Can you work these out from the model? Positions are in its coordinate system, mm. Face numbers are marked on the shaded views. Give positions to 0.01 mm unless a question says otherwise; leave off trailing zeros. Loops run counter-clockwise (first coordinate to the right, second up) from the corner with the lowest first, then second, coordinate; pieces in that order, holes last. Notation, with made-up numbers: M 43.25,1.5 L 91.25,1.5 A31 ccw 91.25,28.5 Z; hole C -39.75,22.25 d6. An arc over 180 degrees is marked long. Answer as a JSON object with one key per item and string values.
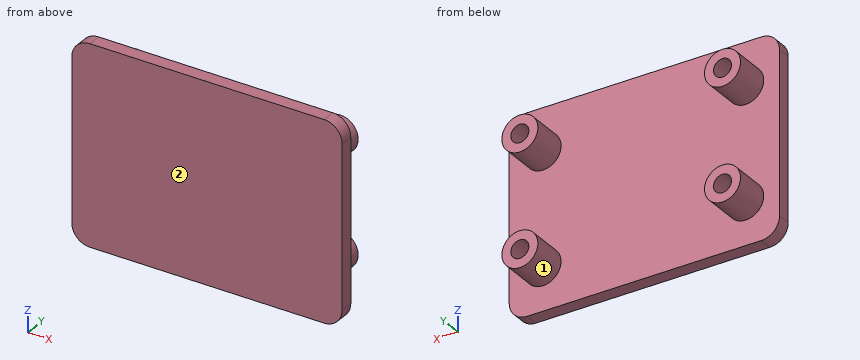
```python
from build123d import *

# Parameters (mm, degrees)
BOSS_EXTRUDE1_DEPTH = 3
SKETCH2_R           = 4
BOSS_EXTRUDE2_DEPTH = 8
SKETCH3_R           = 2
CUT_EXTRUDE1_DEPTH  = 7


with BuildPart() as part:
    # Sketch1 → Boss-Extrude1 (new body)
    with BuildSketch(Plane(origin=(0, 0, 0), x_dir=(1, 0, 0), z_dir=(0, 1, 0))):
        with BuildLine():
            Line((-26, -22), (26, -22))
            ThreePointArc((26, -22), (28.828427125, -20.828427125), (30, -18))
            Line((30, -18), (30, 18))
            ThreePointArc((30, 18), (28.828427125, 20.828427125), (26, 22))
            Line((26, 22), (-26, 22))
            ThreePointArc((-26, 22), (-28.828427125, 20.828427125), (-30, 18))
            Line((-30, 18), (-30, -18))
            ThreePointArc((-30, -18), (-28.828427125, -20.828427125), (-26, -22))
        make_face()
    extrude(amount=BOSS_EXTRUDE1_DEPTH)

    # Sketch2 → Boss-Extrude2 (add)
    with BuildSketch(Plane(origin=(0, 3, 0), x_dir=(1, 0, 0), z_dir=(0, 1, 0))):
        with Locations(Location((22.5, -12.5, 0), (0, 0, 270))):
            Circle(SKETCH2_R)
        with Locations(Location((22.5, 12.5, 0), (0, 0, 270))):
            Circle(SKETCH2_R)
        with Locations(Location((-22.5, -12.5, 0), (0, 0, 270))):
            Circle(SKETCH2_R)
        with Locations(Location((-22.5, 12.5, 0), (0, 0, 270))):
            Circle(SKETCH2_R)
    extrude(amount=BOSS_EXTRUDE2_DEPTH)

    # Sketch3 → Cut-Extrude1 (cut)
    with BuildSketch(Plane(origin=(0, 11, 0), x_dir=(1, 0, 0), z_dir=(0, 1, 0))):
        with Locations(Location((22.5, -12.5, 0), (0, 0, 270))):
            Circle(SKETCH3_R)
        with Locations(Location((22.5, 12.5, 0), (0, 0, 270))):
            Circle(SKETCH3_R)
        with Locations(Location((-22.5, -12.5, 0), (0, 0, 270))):
            Circle(SKETCH3_R)
        with Locations(Location((-22.5, 12.5, 0), (0, 0, 270))):
            Circle(SKETCH3_R)
    extrude(amount=-CUT_EXTRUDE1_DEPTH, mode=Mode.SUBTRACT)


solid = part.part
```
1) Suppose I cut it at D-D, the plane x = -6.5. Write out the boundary of the cut face in (y, z), and give its area (3 significant figures).
Answer list:
{"outline": "M 0,-22 L 3,-22 L 3,22 L 0,22 Z", "area": "132 mm^2"}
2) If we mould it in two halves opening along X, with no side actions, what happens to the marked faces 1 and 2? For each: +X half, -X half, draft (parallel to the pull), parting line (faces both ways), or undercut.
Answer list:
{"face 1": "undercut", "face 2": "draft"}
3) Please list where these lines run through material, in increasing order: line 1 along X through (y, z) = (9.5, 12.5); line 2 along Z through (x, y) = (-21.5, 8.25); line 3 along X through (y, z) = (9.5, 11.5). Write a range as from..to.
Answer list:
{"line 1": "-26.5..-24.5, -20.5..-18.5, 18.5..20.5, 24.5..26.5", "line 2": "-16.37..-14.23, -10.77..-8.63, 8.63..10.77, 14.23..16.37", "line 3": "-26.37..-24.23, -20.77..-18.63, 18.63..20.77, 24.23..26.37"}
4) Suppose I cut it at B-B, the plane x = 22.5. Write out the boundary of the cut face in (y, z).
Answer list:
{"outline": "M 0,-22 L 3,-22 L 3,-16.5 L 11,-16.5 L 11,-14.5 L 4,-14.5 L 4,-10.5 L 11,-10.5 L 11,-8.5 L 3,-8.5 L 3,8.5 L 11,8.5 L 11,10.5 L 4,10.5 L 4,14.5 L 11,14.5 L 11,16.5 L 3,16.5 L 3,22 L 0,22 Z"}
5) Will these pins go through, and if not, where does the flat tip stop? pin 1 Ø4 at (y, z) = (7.5, 16) entering from +X; pin 2 Ø13 at (x, z) = (-5, 10.5) entering from +Y; pin 3 Ø1.2 at (x, z) = (22, 13) entering from +Y.
Answer list:
{"pin 1": "x = 26.21", "pin 2": "y = 3", "pin 3": "y = 4"}
6) Suppose I cut it at A-A, the plane y = 9.75. Write out the boundary of the cut face in (x, z), and give its area (3 significant figures).
Answer list:
{"outline": "C -22.5,-12.5 d8; C -22.5,12.5 d8; C 22.5,-12.5 d8; C 22.5,12.5 d8; hole C -22.5,-12.5 d4; hole C -22.5,12.5 d4; hole C 22.5,-12.5 d4; hole C 22.5,12.5 d4", "area": "151 mm^2"}
7) Suppose I cut it at C-C, the plane z = 12.5. Write out the boundary of the cut face in (x, y).
Answer list:
{"outline": "M -30,0 L 30,0 L 30,3 L 26.5,3 L 26.5,11 L 24.5,11 L 24.5,4 L 20.5,4 L 20.5,11 L 18.5,11 L 18.5,3 L -18.5,3 L -18.5,11 L -20.5,11 L -20.5,4 L -24.5,4 L -24.5,11 L -26.5,11 L -26.5,3 L -30,3 Z"}
